```python
from build123d import *

# Parameters (mm, degrees)
SKETCH1_R           = 6
BOSS_EXTRUDE1_DEPTH = 20
SKETCH2_R           = 2.1
CUT_EXTRUDE1_DEPTH  = 16


with BuildPart() as part:
    # Sketch1 → Boss-Extrude1 (new, symmetric)
    with BuildSketch(Plane.XY):
        Polygon((-26, 20), (-26, -8), (-14, -20), (14, -20), (26, -8), (26, 20), align=None)
        Circle(SKETCH1_R, mode=Mode.SUBTRACT)
    extrude(amount=BOSS_EXTRUDE1_DEPTH, both=True)

    # Sketch2 → Cut-Extrude1 (cut)
    with BuildSketch(Plane(origin=(0, 20, 0), x_dir=(1, 0, 0), z_dir=(0, 1, 0))):
        with Locations(Location((-19.875, 11.875, 0), (0, 0, 270))):
            Circle(SKETCH2_R)
        with Locations(Location((19.875, 11.875, 0), (0, 0, 270))):
            Circle(SKETCH2_R)
        with Locations(Location((19.875, -11.875, 0), (0, 0, 270))):
            Circle(SKETCH2_R)
        with Locations(Location((-19.875, -11.875, 0), (0, 0, 270))):
            Circle(SKETCH2_R)
    extrude(amount=-CUT_EXTRUDE1_DEPTH, mode=Mode.SUBTRACT)


solid = part.part
```
Can you work these out from the model? Positions are in its coordinate system, mm. A direction names the side the tool comes from. Round coordinates to 2 decimals unless told otherwise and drop trailing zeros. Order: outer loops, then holes, each group sorted by start corner. A loop starts at its lowest first (then second) coordinate and runs counter-clockwise, first axis right, second up.
(1) If we section it at C-C (y = 0): Please give me the cut outline in (x, z).
Results are:
outline: (-26, -20) - (-6, -20) - (-6, 20) - (-26, 20) - close; (6, -20) - (26, -20) - (26, 20) - (6, 20) - close
(2) If we section it at D-D (y = 8): Please give me the cut outline in (x, z) (3 decimals), plus the area to 3 significant figures.
Results are:
outline: (-26, -20) - (26, -20) - (26, 20) - (-26, 20) - close; hole circle Ø4.2 at (-19.875, -11.875); hole circle Ø4.2 at (-19.875, 11.875); hole circle Ø4.2 at (19.875, -11.875); hole circle Ø4.2 at (19.875, 11.875)
area: 2,020 mm2
(3) If we section it at A-A (x = 0): Please give me the cut outline in (y, z), plus the area to 3 significant figures.
Results are:
outline: (-20, -20) - (-6, -20) - (-6, 20) - (-20, 20) - close; (6, -20) - (20, -20) - (20, 20) - (6, 20) - close
area: 1,120 mm2
(4) If I drill on L1, parallel to X at y = 14, z = 12; L2, parallel to Y at x = 0, z = 9.5; L3, parallel to X at y = -3.5, z = -8, over which ranges is the centre line in solid material (lowest first)?
Results are:
L1: x = -26 to -21.97, -17.78 to 17.78, 21.97 to 26
L2: y = -20 to -6, 6 to 20
L3: x = -26 to -4.87, 4.87 to 26
(5) We'd pull the mould along X, two halves only. Please class faces 3 (the face through (-6, 0, 0)), 4 (the face through (-26, 6, 0)), 5 (the face through (0, -20, 0)): +X half, -X half, draft (parallel to the pull), parting line (faces both ways), or undercut.
Results are:
face 3: undercut
face 4: -X half
face 5: draft
(6) If we section it at B-B (z = -2): Please give me the cut outline in (x, y).
Results are:
outline: (-26, -8) - (-14, -20) - (14, -20) - (26, -8) - (26, 20) - (-26, 20) - close; hole circle Ø12 at (0, 0)
(7) On a 3-axis mill with a long thin cutter (end or side, diameter ignored), from which of +Z, -Z, +X, -X, +Y, -Y can I reach the whole of each face in a straight line? I mean faces 1 (the face through (-6, 5, 20)), 2 (the face through (-17.793, 12.112, -12.148)). Say none if no direction works.
Results are:
face 1: +Z, +X, -X, +Y, -Y
face 2: +Y
(8) I'm going to push flat-ended pins straight in: pin 1 (2.5 mm diameter, centred on x = -19.875, z = 11.875, fed in from +Y); pin 2 (4.5 mm diameter, centred on x = -20.5, z = 12, fed in from +Y); pin 3 (4 mm diameter, centred on x = 19.875, z = -11.875, fed in from -Y) (3 decimals). Where does each tip first touch, or does it pass through?
Results are:
pin 1: stops at y = 4
pin 2: stops at y = 20
pin 3: stops at y = -16.125
